from build123d import *

# Parameters (mm, degrees)
PAD_DEPTH    = 40
SKETCH001_R  = 3.215442
PAD001_DEPTH = 100
SKETCH002_R  = 1.790301
PAD002_DEPTH = 10
FILLET_R     = 1
FILLET001_R  = 1
CHAMFER_SIZE = 0.2
FILLET002_R  = 2
PAD003_DEPTH = 10
FILLET003_R  = 1
FILLET004_R  = 1


with BuildPart() as part:
    # Sketch → Pad (new body)
    with BuildSketch(Plane.XZ):
        Polygon((2.886751, -5), (5.773503, 0), (2.886751, 5), (-2.886751, 5), (-5.773503, 0), (-2.886751, -5), align=None)
    extrude(amount=PAD_DEPTH)

    # Sketch001 (on Face7 of Pad) → Pad001 (join)
    with BuildSketch(Plane(origin=(0, 0, 0), x_dir=(1, 0, 0), z_dir=(0, 1, 0))):
        Circle(SKETCH001_R)
    extrude(amount=PAD001_DEPTH)

    # Sketch002 (on Face10 of Pad001) → Pad002 (join)
    with BuildSketch(Plane(origin=(0, 100, 0), x_dir=(1, 0, 0), z_dir=(0, 1, 0))):
        Circle(SKETCH002_R)
    extrude(amount=PAD002_DEPTH)

    # Fillet
    fillet_edges = [part.edges().sort_by_distance(p)[0] for p in [
        (-1.790301, 100, 0),
    ]]
    fillet(fillet_edges, radius=FILLET_R)

    # Fillet001
    fillet001_edges = [part.edges().sort_by_distance(p)[0] for p in [
        (-1.790301, 110, 0),
    ]]
    fillet(fillet001_edges, radius=FILLET001_R)

    # Chamfer
    chamfer_edges = [part.edges().sort_by_distance(p)[0] for p in [
        (-3.215442, 100, 0),
    ]]
    chamfer(chamfer_edges, length=CHAMFER_SIZE)

    # Sketch003 → Groove (revolve, cut)
    with BuildSketch(Plane.XY):
        Polygon((3.201163, 0), (6.726055, -29.548664), (6.726055, 0), align=None)
    revolve(axis=Axis((0, 0, 0), (0, 1, 0)), mode=Mode.SUBTRACT)

    # Fillet002
    fillet002_edges = [part.edges().sort_by_distance(p)[0] for p in [
        (4.330127, -40, -2.5),
        (4.330127, -40, 2.5),
        (0, -40, 5),
        (-4.330127, -40, 2.5),
        (-4.330127, -40, -2.5),
        (0, -40, -5),
    ]]
    fillet(fillet002_edges, radius=FILLET002_R)

    # Sketch004 → Pad003 (join)
    with BuildSketch(Plane.XY.offset(2)):
        with BuildLine():
            ThreePointArc((1.577738, 92.233203), (0, 93.810941), (-1.577738, 92.233203))
            Line((-1.577738, 92.233203), (-1.577738, 80.809975))
            ThreePointArc((-1.577738, 80.809975), (0, 79.232237), (1.577738, 80.809975))
            Line((1.577738, 80.809975), (1.577738, 92.233203))
        make_face()
    extrude(amount=PAD003_DEPTH)

    # Fillet003
    fillet003_edges = [part.edges().sort_by_distance(p)[0] for p in [
        (0, 93.810941, 12),
        (-1.577738, 86.521589, 12),
        (0, 79.232237, 12),
        (1.577738, 86.521589, 12),
    ]]
    fillet(fillet003_edges, radius=FILLET003_R)

    # Fillet004
    fillet004_edges = [part.edges().sort_by_distance(p)[0] for p in [
        (-1.577738, 86.521589, 2.801751),
        (0, 79.232237, 3.215442),
        (0, 93.810941, 3.215442),
        (1.577738, 86.521589, 2.801751),
    ]]
    fillet(fillet004_edges, radius=FILLET004_R)


solid = part.part
Work out the finished part from the listing and answer in its coordinate system (mm). A direction names the side the tool comes from. Round coordinates to 2 decimals unless told otherwise and drop trailing zeros. Write each loop counter-clockwise with the first axis right and the second up, starting at its lowest first coordinate (ties: lowest second). Pieces come first, ordered by that corner, then holes. Notation, with made-up numbers: (62, -11) - (84, -11) arc R34 ccw to (84, 24) - close; hole circle Ø6 at (-35.75, -32). An arc over 180 degrees is marked (long way). Answer in a Markdown table with one row per item. Add a question column.
1. Given pin 1 (1.8 mm diameter, centred on x = 1, z = 0.5, fed in from +Y); pin 2 (3 mm diameter, centred on x = -1.5, z = 8.5, fed in from -Y); pin 3 (2.5 mm diameter, centred on y = 84.5, z = 8.5, fed in from -X); pin 4 (6 mm diameter, centred on y = 6.5, z = 3, fed in from +X), each flat-ended and moving along its own axis, determine where each tip first touches the part or whether it passes through.
2. The mould has two halves that part along Y. Classify faces 4 (the cylindrical face through (0.03, 93.81, 7.11)), 5 (the cylindrical face through (-0.419, 49.201, -3.188)), 6 (the flat face through (0, -26, 5)): +Y half, -Y half, draft (parallel to the pull), parting line (faces both ways), or undercut.
3. A cutting plane is placed at A-A, the plane z = 7.75. Determine the outline of the cut face in (x, y), and give its area (3 significant figures).
4. For faces 1 (the flat face through (1.578, 86, 7)), 2 (the cylindrical face through (-0.035, 79.233, 7.114)), 3 (the conical face through (-0.91, -8.54, 4.12)), determine the directions among +Z, -Z, +X, -X, +Y, -Y from which every point of the face is accessible in a straight line to the end or side of a thin tool.
5. A cutting plane is placed at B-B, the plane y = 21. Determine the outline of the cut face in (x, z).
6. Find the intervals of material crossed by line 1 along Y through (x, z) = (0, 6); line 2 along Z through (x, y) = (-1.25, 79); line 3 along Z through (x, y) = (3.75, -17), in increasing order. Write a range as from..to.
Worked out:
| question | item | result |
|---|---|---|
| 1 | pin 1 | y = 110 |
| 1 | pin 2 | y = 79.23 |
| 1 | pin 3 | x = -1.58 |
| 1 | pin 4 | x = 3.22 |
| 2 | face 4 | +Y half |
| 2 | face 5 | undercut |
| 2 | face 6 | draft |
| 3 | outline | (-1.58, 80.81) arc R1.58 ccw to (1.58, 80.81) - (1.58, 92.23) arc R1.58 ccw to (-1.58, 92.23) - close |
| 3 | area | 43.9 mm^2 |
| 4 | face 1 | +Z, +X, +Y |
| 4 | face 2 | +Z |
| 4 | face 3 | none |
| 5 | outline | circle Ø6.43 at (0, 0) |
| 6 | line 1 | 79.23..93.81 |
| 6 | line 2 | -2.96..2.97 |
| 6 | line 3 | -3.5..3.5 |
